The listing builds one solid part. Answer for the finished solid, in the listing's coordinates (mm). A direction names the side the tool comes from. Give positions to 0.01 mm unless a question says otherwise; leave off trailing zeros. Order: outer loops, then holes, each group sorted by start corner. A loop starts at its lowest first (then second) coordinate and runs counter-clockwise, first axis right, second up. Notation, with made-up numbers: (53, 45) - (83, 45) arc R31 cw to (83, 76) - close; hole circle Ø4 at (50, 68.5). An arc over 180 degrees is marked (long way). Answer in a Markdown table with one row per item. Add a question column.
```python
from build123d import *

# Parameters (mm, degrees)
SKETCH1_R           = 3.5
BOSS_EXTRUDE1_DEPTH = 4
CUT_EXTRUDE1_DEPTH  = 2.25
CHAMFER1_SIZE       = 0.35
SKETCH_1_R          = 2
EXTRUDE_1_DEPTH     = 20


with BuildPart() as part:
    # Sketch1 → Boss-Extrude1 (new body)
    with BuildSketch(Plane(origin=(0, 0, 0), x_dir=(1, 0, 0), z_dir=(0, 1, 0))):
        with Locations(Location((0, 0, 0), (0, 0, 270))):
            Circle(SKETCH1_R)
    extrude(amount=BOSS_EXTRUDE1_DEPTH)

    # Sketch2 → Cut-Extrude1 (cut)
    with BuildSketch(Plane(origin=(0, 4, 0), x_dir=(1, 0, 0), z_dir=(0, 1, 0))):
        Polygon((0.866025404, 1.5), (-0.866025404, 1.5), (-1.732050808, 0), (-0.866025404, -1.5), (0.866025404, -1.5), (1.732050808, 0), align=None)
    extrude(amount=-CUT_EXTRUDE1_DEPTH, mode=Mode.SUBTRACT)

    # Cut-Extrude2 cone 1 section (through the dimple's axis) → Cut-Extrude2 (revolve, cut)
    with BuildSketch(Plane(origin=(0, 4, 0), x_dir=(0, 0, 1), z_dir=(1, 0, 0))):
        Polygon((0, 0), (1.732050808, 0), (0, 1.732050808), align=None)
    revolve(axis=Axis((0, 4, 0), (0, -1, 0)), mode=Mode.SUBTRACT)

    # Chamfer1
    chamfer1_edges = [part.edges().sort_by_distance(p)[0] for p in [
        (0, 0, -3.5),
        (0, 4, -3.5),
    ]]
    chamfer(chamfer1_edges, length=CHAMFER1_SIZE)

    # 草图1 → 凸台-拉伸1 (add)
    with BuildSketch(Plane(origin=(0, 0, 0), x_dir=(-1, 0, 0), z_dir=(0, -1, 0))):
        with Locations(Location((0, 0, 0), (0, 0, 90))):
            Circle(SKETCH_1_R)
    extrude(amount=EXTRUDE_1_DEPTH)


solid = part.part
```
(1) For faces 5 (the face through (-1.4, 3.88, -0.8)), 6 (the face through (-2, -10, 0)), 7 (the face through (-1.4, 4, 1.4)), determine the directions among +Z, -Z, +X, -X, +Y, -Y from which every point of the face is accessible in a straight line to the end or side of a thin tool.
(2) Each of these flat-tipped pins is pushed along its axis until it touches: P1, Ø2, axis at x = 1, y = -17, coming from the -Z side; P2, Ø3, axis at x = 0, y = -7.5, coming from the +Z side. Where does it stop, or does it pass through?
(3) The mould has two halves that part along Z. Classify faces 1 (the face through (-1.305, 2.891, 0.74)), 2 (the face through (0, 1.75, 0)), 3 (the face through (-3.417, 1.977, -0.759)), 4 (the face through (0, -20, 0)): +Z half, -Z half, draft (parallel to the pull), parting line (faces both ways), or undercut.
(4) Find section B-B, the plane y = -11. Write down the section's boundary in (x, z), plus the area to 3 significant figures.
(5) Find section A-A, the plane x = 0. Write down the section's boundary in (y, z), plus the area to 3 significant figures.
(6) Straight lines are drawn through the part: line 1 (Y direction, x = -0.25, z = -2.5); line 2 (X direction, y = -2, z = 0); line 3 (X direction, y = -11.25, z = -1). For each, find the intervals that lie inside material, in ascending order.
Answer key:
| question | item | result |
|---|---|---|
| 1 | face 5 | +Y |
| 1 | face 6 | -Y |
| 1 | face 7 | +Z, -Z, +X, -X, +Y |
| 2 | P1 | z = -2 |
| 2 | P2 | z = 2 |
| 3 | face 1 | undercut |
| 3 | face 2 | undercut |
| 3 | face 3 | parting line |
| 3 | face 4 | draft |
| 4 | outline | circle Ø4 at (0, 0) |
| 4 | area | 12.6 mm² |
| 5 | outline | (-20, -2) - (0, -2) - (0, -3.15) - (0.35, -3.5) - (3.65, -3.5) - (4, -3.15) - (4, -1.73) - (3.77, -1.5) - (1.75, -1.5) - (1.75, 1.5) - (3.77, 1.5) - (4, 1.73) - (4, 3.15) - (3.65, 3.5) - (0.35, 3.5) - (0, 3.15) - (0, 2) - (-20, 2) - close |
| 5 | area | 101 mm² |
| 6 | line 1 | 0 to 4 |
| 6 | line 2 | -2 to 2 |
| 6 | line 3 | -1.73 to 1.73 |
